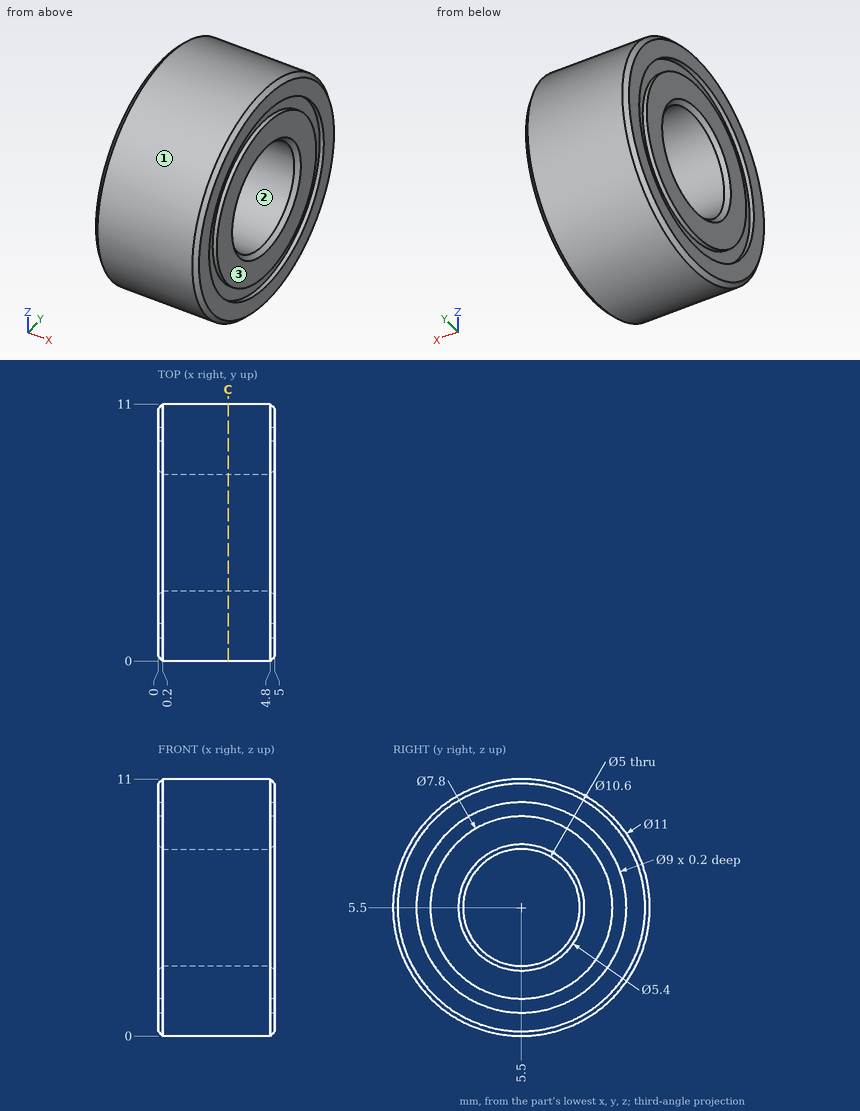
The figure shows three views and two pictorial views of one solid part (mm, origin at its lowest corner). Answer the questions. Give positions to 0.01 mm unless a question says otherwise; leave off trailing zeros. Order: outer loops, then holes, each group sorted by start corner. A loop starts at its lowest first (then second) coordinate and runs counter-clockwise, first axis right, second up. Notation, with made-up numbers: (65, -30.5) - (115, -30.5) arc R23 cw to (115, -5.5) - close; hole circle Ø10 at (21, 73). An arc over 180 degrees is marked (long way). Answer as CSV lines item,"result".
Q1. Determine the mould class of the marked faces 1, 2 and 3 for opening direction Z: pulls with the +Z half, pulls with the -Z half, needs draft (parallel to the pull), parting line crosses it, or undercut.
Answer key:
face 1,"parting line crosses it"
face 2,"undercut"
face 3,"needs draft"
Q2. Straight lines are drawn through the part: L1, parallel to Y at x = 4.7, z = 7.75; L2, parallel to X at y = 2.5, z = 2.75; L3, parallel to Y at x = 1.15, z = 7.25. For each, find the intervals that lie inside material, in ascending order.
Answer key:
L1,"y = 0.48 to 4.41, 6.59 to 10.52"
L2,"x = 0.2 to 4.8"
L3,"y = 0.29 to 3.71, 7.29 to 10.71"
Q3. Each of these flat-tipped pins is pushed along its axis until it touches: pin 1 Ø2 at (x, z) = (3.5, 7.5) entering from -Y; pin 2 Ø5 at (y, z) = (5.5, 5) entering from -X; pin 3 Ø1.5 at (x, y) = (4, 9) entering from -Z. Where does it stop, or does it pass through?
Answer key:
pin 1,"stops at y = 0.09"
pin 2,"stops at x = 0"
pin 3,"stops at z = 0.74"
Q4. A cutting plane is placed at C-C, the plane x = 3. Determine the outline of the cut face in (y, z).
Answer key:
outline,"circle Ø11 at (5.5, 5.5); hole circle Ø5 at (5.5, 5.5)"
